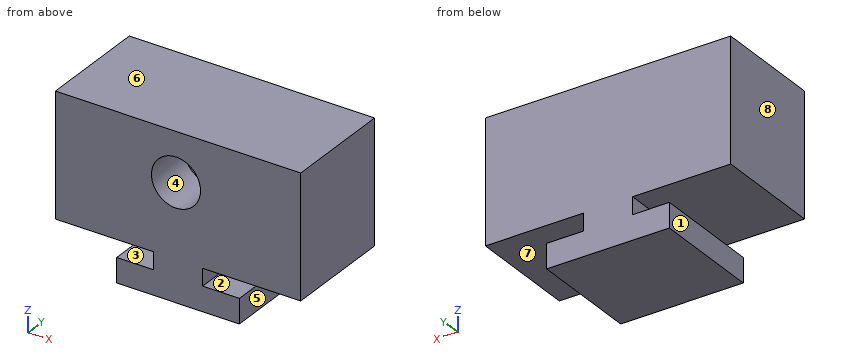
from build123d import *

# Parameters (mm, degrees)
F0_W      = 127
F0_H      = 85.09
F1_DEPTH  = 57.15
F2_W      = 31.75
F2_H      = 12.7
F3_DEPTH  = 57.15
F4_W      = 50.8
F4_H      = 8.89
F5_DEPTH  = 57.15
F6_W      = 31.75
F6_H      = 12.7
F7_DEPTH  = 57.15
F8_W      = 50.8
F8_H      = 8.89
F9_DEPTH  = 57.15
F10_R     = 12.7
F11_DEPTH = 25.4


with BuildPart() as f1:
    # F0 (on Front) → F1 (new body)
    with BuildSketch(Plane.XZ):
        with Locations((63.5, -42.545)):
            Rectangle(F0_W, F0_H)
    extrude(amount=F1_DEPTH)

    # F2 (on face) → F3 (cut)
    with BuildSketch(Plane.XZ.offset(57.15)):
        with Locations((111.125, -78.74)):
            Rectangle(F2_W, F2_H)
    extrude(amount=-F3_DEPTH, mode=Mode.SUBTRACT)

    # F4 (on face) → F5 (cut)
    with BuildSketch(Plane.XZ.offset(57.15)):
        with Locations((101.6, -67.945)):
            Rectangle(F4_W, F4_H)
    extrude(amount=-F5_DEPTH, mode=Mode.SUBTRACT)

    # F6 (on face) → F7 (cut)
    with BuildSketch(Plane.XZ.offset(57.15)):
        with Locations((15.875, -78.74)):
            Rectangle(F6_W, F6_H)
    extrude(amount=-F7_DEPTH, mode=Mode.SUBTRACT)

    # F8 (on face) → F9 (cut)
    with BuildSketch(Plane.XZ.offset(57.15)):
        with Locations((25.4, -67.945)):
            Rectangle(F8_W, F8_H)
    extrude(amount=-F9_DEPTH, mode=Mode.SUBTRACT)

    # F10 (on face) → F11 (cut)
    with BuildSketch(Plane.XZ.offset(57.15)):
        with Locations((62.435351, -25.4)):
            Circle(F10_R)
    extrude(amount=-F11_DEPTH, mode=Mode.SUBTRACT)


solid = f1.part
Input: part model. Units: mm. Frame: model coordinates. Face numbers are marked on the shaded views. A direction names the side the tool comes from. Give positions to 0.01 mm unless a question says otherwise; leave off trailing zeros. Order: outer loops, then holes, each group sorted by start corner. A loop starts at its lowest first (then second) coordinate and runs counter-clockwise, first axis right, second up.
Q1. Section D-D on z = -35. Output: boundary loops of the cut face in (x, y), and give its area (3 significant figures).
Checked values:
outline: (0, -57.15) - (54.12, -57.15) - (54.12, -31.75) - (70.75, -31.75) - (70.75, -57.15) - (127, -57.15) - (127, 0) - (0, 0) - close
area: 6,840 mm2
Q2. Draft query along Z for the marked faces 6, 7 and 8. Return one class per face: +Z half, -Z half, draft (parallel to the pull), parting line (faces both ways), or undercut.
Checked values:
face 6: +Z half
face 7: undercut
face 8: draft
Q3. Section C-C on x = 28.5. Output: boundary loops of the cut face in (y, z), and give its area (3 significant figures).
Checked values:
outline: (-57.15, -63.5) - (0, -63.5) - (0, 0) - (-57.15, 0) - close
area: 3,630 mm2
Q4. Section A-A on y = -41.5. Output: boundary loops of the cut face in (x, z).
Checked values:
outline: (0, -63.5) - (50.8, -63.5) - (50.8, -72.39) - (31.75, -72.39) - (31.75, -85.09) - (95.25, -85.09) - (95.25, -72.39) - (76.2, -72.39) - (76.2, -63.5) - (127, -63.5) - (127, 0) - (0, 0) - close; hole circle Ø25.4 at (62.44, -25.4)
Q5. Ray query, probe 1 along Z at (x, y) = (46.5, -36); probe 2 along Z at (x, y) = (119.5, -26); probe 3 along X at (y, z) = (-7.5, -66.5). Return the intervals inside material, ascending.
Checked values:
probe 1: z = -85.09 to -72.39, -63.5 to 0
probe 2: z = -63.5 to 0
probe 3: x = 50.8 to 76.2
Q6. Section B-B on z = -25.4. Output: boundary loops of the cut face in (x, y), and give its area (3 significant figures).
Checked values:
outline: (0, -57.15) - (49.74, -57.15) - (49.74, -31.75) - (75.14, -31.75) - (75.14, -57.15) - (127, -57.15) - (127, 0) - (0, 0) - close
area: 6,610 mm2
Q7. Contact query for flat-ended pins moving along their axis: pin 1 Ø12.5 at (x, z) = (60.5, -25.5) entering from -Y; pin 2 Ø2.5 at (y, z) = (-37, -68) entering from +X; pin 3 Ø14 at (y, z) = (-19.5, -80) entering from -X. Output: stop coordinate, or through.
Checked values:
pin 1: stops at y = -31.75
pin 2: stops at x = 76.2
pin 3: stops at x = 31.75
Q8. Set-up query: the marked faces 1, 2, 3, 4 and 5. Return all of +Z, -Z, +X, -X, +Y, -Y with unobstructed straight access to the full face (end or side cutting, diameter ignored); none if empty.
Checked values:
face 1: -Z, -X, +Y, -Y
face 2: +X, +Y, -Y
face 3: -X, +Y, -Y
face 4: -Y
face 5: -Z, +X, +Y, -Y
